Check sheet for the modelled part. Datum: model origin and axes. Units: mm. Face numbers are marked on the shaded views. A direction names the side the tool comes from. Coordinates: 2 decimals unless noted, no trailing zeros. Loops run counter-clockwise (first coordinate to the right, second up) from the corner with the lowest first, then second, coordinate; pieces in that order, holes last. Notation, with made-up numbers: (30, -25) - (82, -25) arc R29 cw to (82, 12) - close; hole circle Ø3 at (44.5, 78). An arc over 180 degrees is marked (long way). Write each question's results on one line, items separated by ' | '. Start each with the question number.
1. Cross-section at D-D (z = -5). Record the cut outline in (x, y).
2. Cross-section at C-C (y = 11.5). Record the cut outline in (x, z).
3. Thickness scan on line 1 (Y direction, x = 3, z = 3); line 2 (X direction, y = 17.25, z = -2.5); line 3 (X direction, y = 16.9, z = 2.5). Record the ranges inside material, lowest first. Write a range as [from, to].
4. Cross-section at A-A (x = 0). Record the cut outline in (y, z), and give its area (3 significant figures).
5. Gauge pin test, flat ends, axial feed: P1, Ø3, axis at y = 22.5, z = 1, coming from the +X side; P2, Ø1.5, axis at y = 14, z = 1.5, coming from the -X side; P3, Ø4, axis at x = -2, z = -2, coming from the +Y side. Record the tip position at first contact, or that the pin passes through.
6. Cross-section at B-B (z = 2.25). Record the cut outline in (x, y), and give its area (3 significant figures).
7. Tool access check on the marked faces 4 and 5. Record the directions out of +Z, -Z, +X, -X, +Y, -Y that give a thin tool (end or side, any length) a straight path to the whole face; none if there is none.
8. Draft check along Z on the marked faces 1, 2 and 3. Enter one of: released by +Z, released by -Z, zero draft, split by the parting line, or undercut.
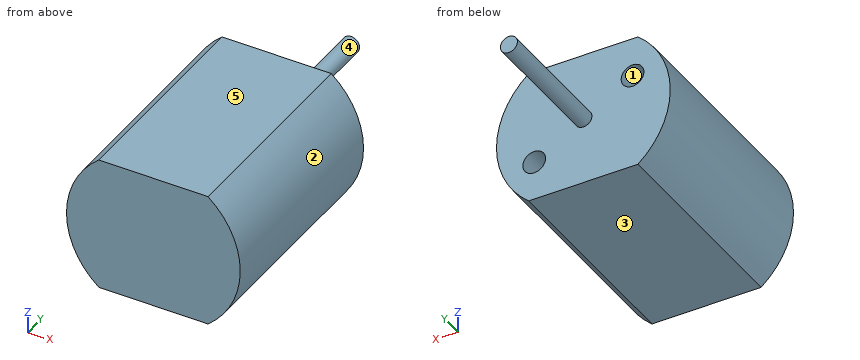
```python
from build123d import *

# Parameters (mm, degrees)
EXTRUDE_1_DEPTH     = 18.7
SKETCH_2_R          = 0.75
EXTRUDE_2_DEPTH     = 11.3
SKETCH_3_R          = 1
CUT_EXTRUDE_1_DEPTH = 3


with BuildPart() as part:
    # 草图1 → 凸台-拉伸1 (new body)
    with BuildSketch(Plane(origin=(0, 0, 0), x_dir=(1, 0, 0), z_dir=(0, 1, 0))):
        with BuildLine():
            Line((4.808326112, 5.95), (-4.808326112, 5.95))
            ThreePointArc((-4.808326112, 5.95), (-7.65, 0), (-4.808326112, -5.95))
            Line((-4.808326112, -5.95), (4.808326112, -5.95))
            ThreePointArc((4.808326112, -5.95), (7.65, 0), (4.808326112, 5.95))
        make_face()
    extrude(amount=EXTRUDE_1_DEPTH)

    # 草图2 → 凸台-拉伸2 (add)
    with BuildSketch(Plane(origin=(0, 18.7, 0), x_dir=(1, 0, 0), z_dir=(0, 1, 0))):
        with Locations(Location((0, 0, 0), (0, 0, 270))):
            Circle(SKETCH_2_R)
    extrude(amount=EXTRUDE_2_DEPTH)

    # 草图3 → 切除-拉伸1 (cut)
    with BuildSketch(Plane(origin=(0, 18.7, 0), x_dir=(1, 0, 0), z_dir=(0, 1, 0))):
        with Locations(Location((4.330127019, 2.5, 0), (0, 0, 270))):
            Circle(SKETCH_3_R)
        with Locations(Location((-4.330127019, -2.5, 0), (0, 0, 270))):
            Circle(SKETCH_3_R)
    extrude(amount=-CUT_EXTRUDE_1_DEPTH, mode=Mode.SUBTRACT)


solid = part.part
```
Established:
1) outline: (-5.79, 0) - (5.79, 0) - (5.79, 18.7) - (-5.79, 18.7) - close
2) outline: (-4.81, -5.95) - (4.81, -5.95) arc R7.65 ccw to (4.81, 5.95) - (-4.81, 5.95) arc R7.65 ccw to start
3) line 1: [0, 18.7] | line 2: [-7.23, 3.33], [5.33, 7.23] | line 3: [-7.23, -5.33], [-3.33, 7.23]
4) outline: (0, -5.95) - (18.7, -5.95) - (18.7, -0.75) - (30, -0.75) - (30, 0.75) - (18.7, 0.75) - (18.7, 5.95) - (0, 5.95) - close | area: 239 mm^2
5) P1: x = 0.75 | P2: x = -7.61 | P3: y = 18.7
6) outline: (-7.31, 0) - (7.31, 0) - (7.31, 18.7) - (-3.36, 18.7) - (-3.36, 15.7) - (-5.3, 15.7) - (-5.3, 18.7) - (-7.31, 18.7) - close | area: 268 mm^2
7) face 4: +Y | face 5: +Z, +X, -X, +Y, -Y
8) face 1: undercut | face 2: split by the parting line | face 3: released by -Z
